Here's how the part is built. I have some questions about the finished solid (model axes, mm). A direction names the side the tool comes from. Give positions to 0.01 mm unless a question says otherwise; leave off trailing zeros. Write each loop counter-clockwise with the first axis right and the second up, starting at its lowest first coordinate (ties: lowest second). Pieces come first, ordered by that corner, then holes. Notation, with made-up numbers: (87.5, 59.5) - (143.5, 59.5) arc R17 ccw to (143.5, 90.5) - close; hole circle Ø3 at (55.5, -28.75). An arc over 180 degrees is marked (long way). Use a Markdown table: item, result.
```python
from build123d import *

# Parameters (mm, degrees)
SKETCH1_W           = 76.2
SKETCH1_H           = 60
BOSS_EXTRUDE1_DEPTH = 2.5
SKETCH2_W           = 15
SKETCH2_H           = 10
BOSS_EXTRUDE2_DEPTH = 2.5
CUT_EXTRUDE1_DEPTH  = 10
FILLET1_R           = 10
FILLET2_R           = 5
FILLET3_R           = 1


with BuildPart() as part:
    # Sketch1 → Boss-Extrude1 (new, symmetric)
    with BuildSketch(Plane(origin=(0, 0, 0), x_dir=(1, 0, 0), z_dir=(0, 1, 0))):
        Rectangle(SKETCH1_W, SKETCH1_H)
    extrude(amount=BOSS_EXTRUDE1_DEPTH, both=True)

    # Sketch2 → Boss-Extrude2 (add, symmetric)
    with BuildSketch(Plane(origin=(0, 0, 0), x_dir=(1, 0, 0), z_dir=(0, 1, 0))):
        with Locations((-45.6, 0)):
            Rectangle(SKETCH2_W, SKETCH2_H)
    boss_extrude2 = extrude(amount=BOSS_EXTRUDE2_DEPTH, both=True)

    # Sketch3 → Cut-Extrude1 (cut)
    with BuildSketch(Plane(origin=(0, 2.5, 0), x_dir=(1, 0, 0), z_dir=(0, 1, 0))):
        with BuildLine():
            Line((-48.1, 2.7), (-40.8, 2.7))
            ThreePointArc((-40.8, 2.7), (-38.1, 0), (-40.8, -2.7))
            Line((-40.8, -2.7), (-48.1, -2.7))
            ThreePointArc((-48.1, -2.7), (-50.8, 0), (-48.1, 2.7))
        make_face()
    cut_extrude1 = extrude(amount=-CUT_EXTRUDE1_DEPTH, mode=Mode.SUBTRACT)

    # Mirror4: Boss-Extrude2, Cut-Extrude1 across plane
    add(boss_extrude2.mirror(Plane(origin=(0, 0, 0), x_dir=(0, 0, 1), z_dir=(1, 0, 0))))
    add(cut_extrude1.mirror(Plane(origin=(0, 0, 0), x_dir=(0, 0, 1), z_dir=(1, 0, 0))), mode=Mode.SUBTRACT)

    # Fillet1
    fillet1_edges = [part.edges().sort_by_distance(p)[0] for p in [
        (-38.1, 0, 5),
        (-38.1, 0, -5),
        (38.1, 0, -5),
        (38.1, 0, 5),
    ]]
    fillet(fillet1_edges, radius=FILLET1_R)

    # Fillet2
    fillet2_edges = [part.edges().sort_by_distance(p)[0] for p in [
        (-53.1, 0, -5),
        (-53.1, 0, 5),
        (53.1, 0, -5),
        (53.1, 0, 5),
    ]]
    fillet(fillet2_edges, radius=FILLET2_R - 0.0001)  # a hair under: the kernel refuses the full size

    # Fillet3
    fillet3_edges = [part.edges().sort_by_distance(p)[0] for p in [
        (38.1, 2.5, 22.5),
        (-51.635563195, 2.5, 3.535563195),
        (-51.635563195, 2.5, -3.535563195),
        (51.635563195, 2.5, 3.535563195),
        (51.635563195, 2.5, -3.535563195),
        (0, 2.5, -30),
        (-38.1, 2.5, -22.5),
        (0, 2.5, 30),
        (38.1, 2.5, -22.5),
        (-38.1, 2.5, 22.5),
        (41.028932188, 2.5, -7.928932188),
        (41.028932188, 2.5, 7.928932188),
        (-41.028932188, 2.5, -7.928932188),
        (-41.028932188, 2.5, 7.928932188),
    ]]
    fillet(fillet3_edges, radius=FILLET3_R)


solid = part.part
```
Item 1: For faces 1 (the cylindrical face through (38.1, 0, -0.1)), 2 (the flat face through (-38.1, 0, -22)), 3 (the flat face through (38.1, 0, 23)), 4 (the cylindrical face through (41.11, -0.53, -7.85)), 5 (the flat face through (-38.1, 0, 23)), which set-ups out of +Z, -Z, +X, -X, +Y, -Y let a thin tool reach every point of the face, with its end or its side?
Values:
| item | result |
|---|---|
| face 1 | +Y, -Y |
| face 2 | -Z, -X, +Y, -Y |
| face 3 | +Z, +X, +Y, -Y |
| face 4 | -Z, +X, +Y, -Y |
| face 5 | +Z, -X, +Y, -Y |
Item 2: If we section it at A-A, the plane y = 0.65: Count the separate pieces of the cut face and the enclosed holes in it, plus the area to 3 significant figures.
Values:
| item | result |
|---|---|
| separate pieces | 1 |
| enclosed holes | 2 |
| area | 4,810 mm2 |
Item 3: If we section it at B-B, the plane z = -22.5: Write out the boundary of the cut face in (x, y), plus the area to 3 significant figures.
Values:
| item | result |
|---|---|
| outline | (-38.1, -2.5) - (38.1, -2.5) - (38.1, 1.5) arc R1 ccw to (37.1, 2.5) - (-37.1, 2.5) arc R1 ccw to (-38.1, 1.5) - close |
| area | 381 mm2 |
Item 4: Thinking about a two-plate mould opening in Z: for faces 6 (the cylindrical face through (-50.8, 0, 0.1)), 7 (the flat face through (38.1, 0, -22)), 8 (the flat face through (-44, 0, 2.7)), 9 (the cylindrical face through (51.67, -0.53, -3.5)), which applies, +Z half, -Z half, draft (parallel to the pull), parting line (faces both ways), or undercut?
Values:
| item | result |
|---|---|
| face 6 | undercut |
| face 7 | draft |
| face 8 | undercut |
| face 9 | -Z half |
Item 5: Will these pins go through, and if not, where does the flat tip stop? pin 1 Ø3 at (y, z) = (0, 19) entering from +X; pin 2 Ø2 at (y, z) = (0.5, 25.5) entering from -X; pin 3 Ø1.5 at (x, y) = (-46, 1) entering from -Z.
Values:
| item | result |
|---|---|
| pin 1 | stops at x = 38.1 |
| pin 2 | stops at x = -38.1 |
| pin 3 | stops at z = -5.41 |
Item 6: I need wall thicknesses on line 1 along X through (y, z) = (-2.2, 1); line 2 along X through (y, z) = (-1.2, 24.5); line 3 along Z through (x, y) = (-39, -0.25). Which ranges of each line are inside material? Lowest first, please. Write a range as [from, to].
Values:
| item | result |
|---|---|
| line 1 | x = [-53, -50.61], [-38.29, 38.29], [50.61, 53] |
| line 2 | x = [-38.1, 38.1] |
| line 3 | z = [-10.85, -2.01], [2.01, 10.85] |
